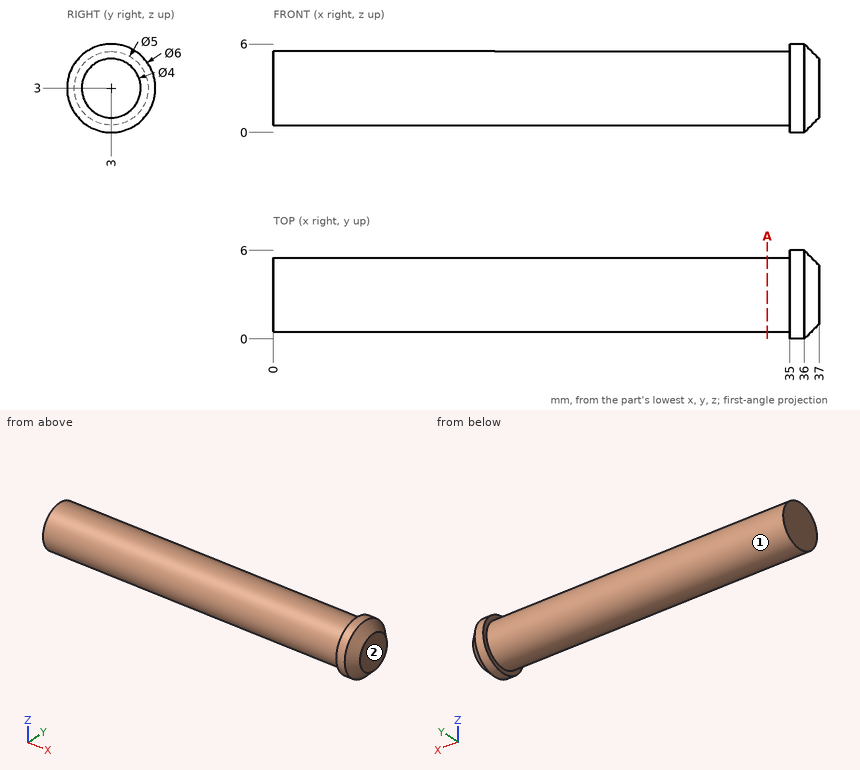
Can you work these out from the drawing? Everything is in mm from the part's minimum corner. A direction names the side the tool comes from. Give positions to 0.01 mm unless a question says otherwise; leave off trailing zeros. Loops run counter-clockwise (first coordinate to the right, second up) from the corner with the lowest first, then second, coordinate; pieces in that order, holes last. Notation, with made-up numbers: (-10.5, -13.75) -> (35.5, -13.75) arc R15 cw to (35.5, 4.25) -> close; hole circle Ø7 at (14, 35.25). An arc over 180 degrees is marked (long way). Return JSON: item names as keys, results as strings.
Q1. I need wall thicknesses on probe 1 along Z at (x, y) = (16, 2.8); probe 2 along Z at (x, y) = (17, 4.5); probe 3 along Y at (x, z) = (12.5, 4.45). Which ranges of each line are inside material? Lowest first, please.
Checks:
{"probe 1": "z = 0.51 to 5.49", "probe 2": "z = 1 to 5", "probe 3": "y = 0.96 to 5.04"}
Q2. On a 3-axis mill with a long thin cutter (end or side, diameter ignored), from which of +Z, -Z, +X, -X, +Y, -Y can I reach the whole of each face in a straight line? I mean the marked faces 1 and 2. Say none if no direction works.
Checks:
{"face 1": "-X", "face 2": "+Z, -Z, +X, +Y, -Y"}
Q3. For pin 1 Ø3 at (x, z) = (6, 2) entering from +Y; pin 2 Ø1.5 at (y, z) = (3.5, 3) entering from -X; pin 3 Ø1 at (x, z) = (11, 4.5) entering from -Y, each with a flat end and sliding along its axis, tell me the tip position at first contact or that it passes through.
Checks:
{"pin 1": "stops at y = 5.5", "pin 2": "stops at x = 0", "pin 3": "stops at y = 0.71"}
Q4. I want a section at A-A, the plane x = 33.5. List the corners of the cut face in (y, z) for me, then the cut area to 3 significant figures.
Checks:
{"outline": "circle Ø5 at (3, 3)", "area": "19.6 mm2"}
